Part model, mm, in its own coordinate system. Face numbers are marked on the shaded views. Round coordinates to 2 decimals unless told otherwise and drop trailing zeros. Loops run counter-clockwise (first coordinate to the right, second up) from the corner with the lowest first, then second, coordinate; pieces in that order, holes last.
(1) Mould opens along X. For the marked faces 1, 2 and 3 say: +X half, -X half, draft (parallel to the pull), parting line (faces both ways), or undercut.
(2) Probe probe 1 along X at (y, z) = (3.45, 27.5); probe 2 along Z at (x, y) = (-20, 3.5); probe 3 along Z at (x, y) = (39.6, 3.4). List the from-to ranges inside material, lowest first.
(3) Cut at C-C on z = 0. List the corners of the cut face in (x, y).
(4) Cut at A-A on x = -6. List the corners of the cut face in (y, z).
(5) Cut at D-D on x = 39.6. List the corners of the cut face in (y, z), then the cut area to 3 significant figures.
(6) Cut at B-B on y = 20. List the corners of the cut face in (x, z), then the cut area to 3 significant figures.
(7) Flat gauge pins, fed straight in: pin 1 (3.5 mm diameter, centred on x = 1.5, z = 0, fed in from +Y); pin 2 (2.5 mm diameter, centred on x = -47, y = 15, fed in from +Z); pin 3 (5 mm diameter, centred on y = 17, z = -22, fed in from -X). Where does each tip first touch, or does it go through?
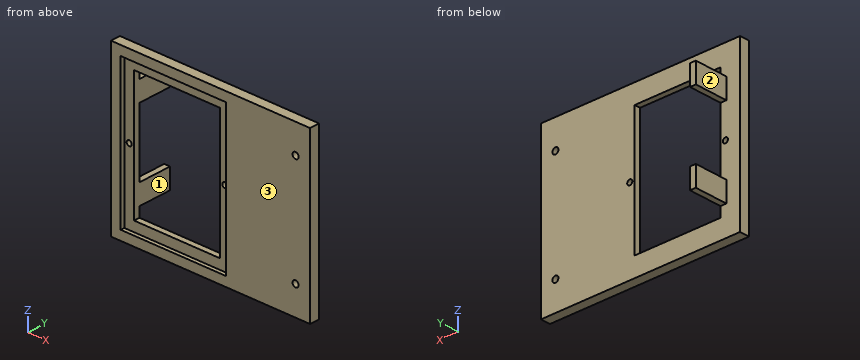
from build123d import *

# Parameters (mm, degrees)
SKETCH1_W           = 110
SKETCH1_H           = 84
BOSS_EXTRUDE1_DEPTH = 5
SKETCH2_W           = 44
SKETCH2_H           = 64.5
CUT_EXTRUDE1_DEPTH  = 5
SKETCH3_R           = 1.55
CUT_EXTRUDE2_DEPTH  = 5
SKETCH5_W           = 3
SKETCH5_H           = 10.213632632
BOSS_EXTRUDE2_DEPTH = 17
SKETCH6_W           = 54
SKETCH6_H           = 74.5
CUT_EXTRUDE3_DEPTH  = 2
CUT_EXTRUDE4_REACH  = 22
SKETCH7_R           = 1.3
SKETCH8_W           = 84
SKETCH8_H           = 5
CUT_EXTRUDE5_DEPTH  = 8


with BuildPart() as part:
    # Sketch1 → Boss-Extrude1 (new body)
    with BuildSketch(Plane(origin=(0, 0, 0), x_dir=(1, 0, 0), z_dir=(0, 1, 0))):
        Rectangle(SKETCH1_W, SKETCH1_H)
    extrude(amount=BOSS_EXTRUDE1_DEPTH)

    # Sketch2 → Cut-Extrude1 (cut)
    with BuildSketch(Plane(origin=(0, 5, 0), x_dir=(1, 0, 0), z_dir=(0, 1, 0))):
        with Locations((-23, 0)):
            Rectangle(SKETCH2_W, SKETCH2_H)
    extrude(amount=-CUT_EXTRUDE1_DEPTH, mode=Mode.SUBTRACT)

    # Sketch3 → Cut-Extrude2 (cut)
    with BuildSketch(Plane(origin=(0, 5, 0), x_dir=(1, 0, 0), z_dir=(0, 1, 0))):
        with Locations((39.6, 27.5)):
            Circle(SKETCH3_R)
        with Locations((39.6, -27.5)):
            Circle(SKETCH3_R)
    extrude(amount=-CUT_EXTRUDE2_DEPTH, mode=Mode.SUBTRACT)

    # Sketch5 → Boss-Extrude2 (add)
    with BuildSketch(Plane(origin=(0, 5, 0), x_dir=(1, 0, 0), z_dir=(0, 1, 0))):
        with Locations((-46.5, 22.143183684)):
            Rectangle(SKETCH5_W, SKETCH5_H)
        with Locations((-46.5, -22.143183684)):
            Rectangle(SKETCH5_W, SKETCH5_H)
    extrude(amount=BOSS_EXTRUDE2_DEPTH)

    # Sketch6 → Cut-Extrude3 (cut)
    with BuildSketch(Plane.XZ):
        with Locations((-23, 0)):
            Rectangle(SKETCH6_W, SKETCH6_H)
    extrude(amount=-CUT_EXTRUDE3_DEPTH, mode=Mode.SUBTRACT)

    # Sketch7 → Cut-Extrude4 (cut, up to next)
    with BuildSketch(Plane.XZ.offset(-2), mode=Mode.PRIVATE) as cut_extrude4_sk1:
        with Locations((-47.5, 0)):
            Circle(SKETCH7_R)
    cut_extrude4_tool1 = extrude(cut_extrude4_sk1.sketch, amount=-CUT_EXTRUDE4_REACH, mode=Mode.PRIVATE) & part.part
    add(cut_extrude4_tool1.solids().sort_by_distance((-47.5, 2, 0))[0], mode=Mode.SUBTRACT)
    # Sketch7 → Cut-Extrude4 (cut, up to next)
    with BuildSketch(Plane.XZ.offset(-2), mode=Mode.PRIVATE) as cut_extrude4_sk2:
        with Locations((1.5, 0)):
            Circle(SKETCH7_R)
    cut_extrude4_tool2 = extrude(cut_extrude4_sk2.sketch, amount=-CUT_EXTRUDE4_REACH, mode=Mode.PRIVATE) & part.part
    add(cut_extrude4_tool2.solids().sort_by_distance((1.5, 2, 0))[0], mode=Mode.SUBTRACT)

    # Sketch8 → Cut-Extrude5 (cut)
    with BuildSketch(Plane(origin=(55, 0, 0), x_dir=(0, 0, -1), z_dir=(1, 0, 0))):
        with Locations((0, 2.5)):
            Rectangle(SKETCH8_W, SKETCH8_H)
    extrude(amount=-CUT_EXTRUDE5_DEPTH, mode=Mode.SUBTRACT)


solid = part.part
Final values:
1. face 1: undercut
1. face 2: -X half
1. face 3: draft
2. probe 1: x = -55 to -45, -1 to 38.05, 41.15 to 47
2. probe 2: z = -42 to -32.25, 32.25 to 42
2. probe 3: z = -42 to -29.05, -25.95 to 25.95, 29.05 to 42
3. outline: (-55, 0) - (-50, 0) - (-50, 2) - (-48.8, 2) - (-48.8, 5) - (-55, 5) - close; (-46.2, 2) - (-45, 2) - (-45, 5) - (-46.2, 5) - close; (-1, 2) - (0.2, 2) - (0.2, 5) - (-1, 5) - close; (2.8, 2) - (4, 2) - (4, 0) - (47, 0) - (47, 5) - (2.8, 5) - close
4. outline: (0, -42) - (5, -42) - (5, -32.25) - (2, -32.25) - (2, -37.25) - (0, -37.25) - close; (0, 37.25) - (2, 37.25) - (2, 32.25) - (5, 32.25) - (5, 42) - (0, 42) - close
5. outline: (0, -42) - (5, -42) - (5, -29.05) - (0, -29.05) - close; (0, -25.95) - (5, -25.95) - (5, 25.95) - (0, 25.95) - close; (0, 29.05) - (5, 29.05) - (5, 42) - (0, 42) - close
5. area: 389 mm2
6. outline: (-48, -27.25) - (-45, -27.25) - (-45, -17.04) - (-48, -17.04) - close; (-48, 17.04) - (-45, 17.04) - (-45, 27.25) - (-48, 27.25) - close
6. area: 61.3 mm2
7. pin 1: stops at y = 5
7. pin 2: stops at z = 27.25
7. pin 3: stops at x = -48
